```python
from build123d import *

# Parameters (mm, degrees)
F1_DEPTH = 25.4
F2_DEPTH = 12.7


with BuildPart() as f1:
    # F0 (on Right) → F1 (new body)
    with BuildSketch(Plane.YZ):
        Polygon((25.4, 0), (0, 0), (0, -31.75), (57.15, -31.75), (57.15, -19.05), align=None)
    extrude(amount=F1_DEPTH)

    # F1_face (on face) → F2 (join)
    with BuildSketch(Plane(origin=(25.4, 24.976667, -17.78), x_dir=(0, 1, 0), z_dir=(1, 0, 0))):
        Polygon((0.423333, 17.78), (-24.976667, 17.78), (-24.976667, -13.97), (32.173333, -13.97), (32.173333, -1.27), align=None)
    extrude(amount=F2_DEPTH)


solid = f1.part
```
Part model, mm, in its own coordinate system. Round coordinates to 2 decimals unless told otherwise and drop trailing zeros. Write each loop counter-clockwise with the first axis right and the second up, starting at its lowest first coordinate (ties: lowest second). Pieces come first, ordered by that corner, then holes. Notation, with made-up numbers: (38, 63.5) -> (42, 63.5) arc R22 ccw to (42, 93.5) -> close; hole circle Ø3 at (-33, -29). An arc over 180 degrees is marked (long way). Return JSON: item names as keys, results as strings. Group by question number.
Q1. Probe L1, parallel to Z at x = 33, y = 54; L2, parallel to Z at x = 22.5, y = 35; L3, parallel to Y at x = 26, z = -8. List the from-to ranges inside material, lowest first. Write a range as [from, to].
Q2. Saw through at B-B on y = 28.5. Write the cut outline in (x, z), plus the area to 3 significant figures.
Q3. Pin check, flat tips, straight feed: pin 1 (12 mm diameter, centred on x = 22, y = 32.5, fed in from +Z); pin 2 (4 mm diameter, centred on x = 7.5, z = -8, fed in from +Y). Stop position of each tip, or through.
Q4. Saw through at A-A on x = 4. Write the cut outline in (y, z).
Q5. Saw through at C-C on z = -6. Write the cut outline in (x, y).
Answer:
{
 "1": {"L1": "[-31.75, -17.16]", "L2": "[-31.75, -5.76]", "L3": "[0, 38.73]"},
 "2": {"outline": "(0, -31.75) -> (38.1, -31.75) -> (38.1, -1.86) -> (0, -1.86) -> close", "area": "1,140 mm2"},
 "3": {"pin 1": "z = -0.66", "pin 2": "y = 42.07"},
 "4": {"outline": "(0, -31.75) -> (57.15, -31.75) -> (57.15, -19.05) -> (25.4, 0) -> (0, 0) -> close"},
 "5": {"outline": "(0, 0) -> (38.1, 0) -> (38.1, 35.4) -> (0, 35.4) -> close"}
}
